```python
from build123d import *

# Parameters (mm, degrees)
SKETCH1_W           = 45.5
SKETCH1_H           = 25.5
SKETCH1_R           = 2.4
BOSS_EXTRUDE1_DEPTH = 15
FILLET1_R           = 2


with BuildPart() as part:
    # Sketch1 → Boss-Extrude1 (new, symmetric)
    with BuildSketch(Plane.XY):
        Rectangle(SKETCH1_W, SKETCH1_H)
        with Locations((-15.426369863, 0)):
            Circle(SKETCH1_R, mode=Mode.SUBTRACT)
        with Locations(Location((15.426369863, 0, 0), (0, 0, 180))):
            Circle(SKETCH1_R, mode=Mode.SUBTRACT)
    extrude(amount=BOSS_EXTRUDE1_DEPTH, both=True)

    # Fillet1
    fillet1_edges = [part.edges().sort_by_distance(p)[0] for p in [
        (-22.75, 12.75, 0),
        (22.75, 12.75, 0),
        (22.75, -12.75, 0),
        (-22.75, -12.75, 0),
    ]]
    fillet(fillet1_edges, radius=FILLET1_R)


solid = part.part
```
The listing builds one solid part. Answer for the finished solid, in the listing's coordinates (mm). Give positions to 0.01 mm unless a question says otherwise; leave off trailing zeros. Order: outer loops, then holes, each group sorted by start corner. A loop starts at its lowest first (then second) coordinate and runs counter-clockwise, first axis right, second up.
Item 1: Given pin 1 Ø4.5 at (x, y) = (-15.43, 0) entering from -Z, flat-ended and moving along its own axis, determine where the tip first touches the part or whether it passes through.
From the geometry:
pin 1: passes through
Item 2: The part is cut by section B-B, the plane z = 8.75. Give the vertices of the cut face in (x, y).
From the geometry:
outline: (-22.75, -10.75) arc R2 ccw to (-20.75, -12.75) - (20.75, -12.75) arc R2 ccw to (22.75, -10.75) - (22.75, 10.75) arc R2 ccw to (20.75, 12.75) - (-20.75, 12.75) arc R2 ccw to (-22.75, 10.75) - close; hole circle Ø4.8 at (-15.43, 0); hole circle Ø4.8 at (15.43, 0)
Item 3: The part is cut by section A-A, the plane y = 0. Give the vertices of the cut face in (x, z).
From the geometry:
outline: (-22.75, -15) - (-17.83, -15) - (-17.83, 15) - (-22.75, 15) - close; (-13.03, -15) - (13.03, -15) - (13.03, 15) - (-13.03, 15) - close; (17.83, -15) - (22.75, -15) - (22.75, 15) - (17.83, 15) - close
Item 4: The part is cut by section C-C, the plane x = -16.5. Give the vertices of the cut face in (y, z), and give its area (3 significant figures).
From the geometry:
outline: (-12.75, -15) - (-2.15, -15) - (-2.15, 15) - (-12.75, 15) - close; (2.15, -15) - (12.75, -15) - (12.75, 15) - (2.15, 15) - close
area: 636 mm2
Item 5: For a pull along X with two mould halves and no side action, classify faces 1 (the face through (17.824, -0.106, -0.21)), 2 (the face through (22.75, 0, 0)), 3 (the face through (-22.18, -12.15, 0.21)) as pulls with the +X half, pulls with the -X half, needs draft (parallel to the pull), parting line crosses it, or undercut.
From the geometry:
face 1: undercut
face 2: pulls with the +X half
face 3: pulls with the -X half
Item 6: Find the intervals of material crossed by probe 1 along X at (y, z) = (-1.25, 13); probe 2 along X at (y, z) = (0.25, -8.25); probe 3 along Y at (x, z) = (-15.5, 11.25), in increasing order.
From the geometry:
probe 1: x = -22.75 to -17.48, -13.38 to 13.38, 17.48 to 22.75
probe 2: x = -22.75 to -17.81, -13.04 to 13.04, 17.81 to 22.75
probe 3: y = -12.75 to -2.4, 2.4 to 12.75
